For this review, take the finished solid that the model builds, in its own axes (mm). Face numbers are marked on the shaded views. Give positions to 0.01 mm unless a question says otherwise; leave off trailing zeros. Order: outer loops, then holes, each group sorted by start corner. A loop starts at its lowest first (then second) coordinate and runs counter-clockwise, first axis right, second up.
from build123d import *

# Parameters (mm, degrees)
BOSS_EXTRUDE1_DEPTH = 27
SKETCH2_R           = 36
CUT_EXTRUDE1_DEPTH  = 54
CHAMFER1_SIZE       = 7
CHAMFER1_SIZE2      = 12.124355653
CHAMFER2_SIZE       = 7
CHAMFER2_SIZE2      = 12.124355653
FILLET1_R           = 2


with BuildPart() as part:
    # Sketch1 → Boss-Extrude1 (new body, symmetric)
    with BuildSketch(Plane.XY):
        Polygon((302.95878724, 482.984033971), (300.611268609, 385.012154555), (321.60524277, 384.509114849), (321.126157335, 364.514853743), (288.135626511, 365.305344711), (288.614711888, 385.299603421), (290.962230577, 483.271485232), align=None)
    extrude(amount=BOSS_EXTRUDE1_DEPTH, both=True)

    # Sketch2 → Cut-Extrude1 (cut)
    with BuildSketch(Plane(origin=(8.913446831, 371.99582848, 0), x_dir=(0.999713055, -0.023954272, 0), z_dir=(-0.023954272, -0.999713055, 0))):
        with Locations((340.302324012, 0)):
            Circle(SKETCH2_R)
    extrude(amount=-CUT_EXTRUDE1_DEPTH, mode=Mode.SUBTRACT)

    # Chamfer1
    chamfer1_edges = [part.edges().sort_by_distance(p)[0] for p in [
        (301.785027925, 433.998094263, 27),
    ]]
    chamfer1_side = [part.faces().sort_by_distance(p)[0] for p in [
        (299.052126571, 412.848339787, 27),
    ]]
    chamfer(chamfer1_edges, length=CHAMFER1_SIZE, length2=CHAMFER1_SIZE2, reference=chamfer1_side[0])

    # Chamfer2
    chamfer2_edges = [part.edges().sort_by_distance(p)[0] for p in [
        (301.785027925, 433.998094263, -27),
    ]]
    chamfer2_side = [part.faces().sort_by_distance(p)[0] for p in [
        (299.052126571, 412.848339787, -27),
    ]]
    chamfer(chamfer2_edges, length=CHAMFER2_SIZE, length2=CHAMFER2_SIZE2, reference=chamfer2_side[0])

    # Fillet1
    fillet1_edges = [part.edges().sort_by_distance(p)[0] for p in [
        (321.126157335, 364.514853743, -24.813708499),
        (288.135626511, 365.305344711, 0),
        (290.962230577, 483.271485232, 0),
        (304.630891923, 364.910099227, -27),
        (321.126157335, 364.514853743, 24.813708499),
        (313.128452892, 364.706487917, 0),
        (313.607538327, 384.700749023, 0),
        (299.459791547, 483.067873922, 20.937822174),
        (302.95878724, 482.984033971, 0),
        (299.459791547, 483.067873922, -20.937822174),
        (304.630891923, 364.910099227, 27),
        (293.461513215, 483.211599553, -27),
        (293.461513215, 483.211599553, 27),
    ]]
    fillet(fillet1_edges, radius=FILLET1_R)


solid = part.part
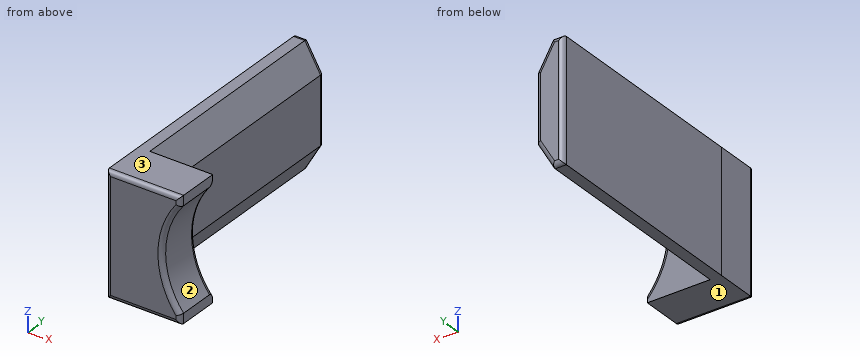
1) We need section A-A on y = 394.5. Give the boundary of the cut face in (x, z).
Answer sheet:
outline: (288.84, -27) - (293.84, -27) - (300.84, -14.88) - (300.84, 14.88) - (293.84, 27) - (288.84, 27) - close
2) Draft analysis for pull direction Z (two halves, no side actions). For the marked faces 1, 2 and 3, state which applies: +Z half, -Z half, draft (parallel to the pull), parting line (faces both ways), or undercut.
Answer sheet:
face 1: -Z half
face 2: undercut
face 3: +Z half
3) To check wall thickness, follow line 1 (Y direction, x = 312.5, z = -6.5); line 2 (Y direction, x = 303, z = 18.5); line 3 (X direction, y = 441.5, z = 9). State the ranges of each line that lie inside material, in increasing order.
Answer sheet:
line 1: y = 364.89 to 384.7
line 2: y = 364.95 to 384.95
line 3: x = 289.96 to 301.96
4) Clearance check with flat-ended pins moving along their axes: pin 1 (12 mm diameter, centred on x = 318, z = -13, fed in from +Y); pin 2 (3 mm diameter, centred on y = 399, z = 4, fed in from -X); pin 3 (5 mm diameter, centred on x = 303, z = -0.5, fed in from -Y). State where each tip first meets the part, or that it passes through.
Answer sheet:
pin 1: stops at y = 384.74
pin 2: stops at x = 288.91
pin 3: stops at y = 364.89
